from build123d import *

# Parameters (mm, degrees)
F0_W     = 1422.4
F0_H     = 50.8
F1_DEPTH = 50.8
F2_T     = -2.54


with BuildPart() as f1:
    # F0 (on Right) → F1 (new body)
    with BuildSketch(Plane.YZ):
        Rectangle(F0_W, F0_H)
    extrude(amount=F1_DEPTH)

    # F2
    f2_openings = [f1.faces().sort_by_distance(p)[0] for p in [
        (25.4, 711.2, 0),
        (25.4, -711.2, 0),
    ]]
    offset(amount=F2_T, openings=f2_openings)


solid = f1.part
Geometry: final body of the model. Coordinates: model frame, mm. A direction names the side the tool comes from. Coordinates: 2 decimals unless noted, no trailing zeros. Order: outer loops, then holes, each group sorted by start corner. A loop starts at its lowest first (then second) coordinate and runs counter-clockwise, first axis right, second up.
(1) Section query C-C (y = 340). Return the cut outline in (x, z), plus the area to 3 significant figures.
(2) Section query B-B (x = 39.5). Return the cut outline in (y, z), plus the area to 3 significant figures.
(3) First-contact query: pin 1 (6 mm diameter, centred on y = 24.5, z = 4.5, fed in from -X). Flat tip, straight axial feed; report the tip coordinate or a pass-through.
(4) Section query A-A (z = -9). Return the cut outline in (x, y).
(5) Draft query along Z for faces 3 (the face through (25, -10, 25.4)), 4 (the face through (25, -10, -25.4)), 5 (the face through (0, -10, 0)), 6 (the face through (48.26, -10, 0)). Return one class per face: pulls with the +Z half, pulls with the -Z half, needs draft (parallel to the pull), parting line crosses it, or undercut.
(6) Material intervals for probe 1 along X at (y, z) = (-635.5, -11); probe 2 along Z at (x, y) = (5, -48), sorted ascending.
(7) Access query for faces 1 (the face through (50.8, -10, 0)), 2 (the face through (25, -10, -22.86)). Directions: +Z, -Z, +X, -X, +Y, -Y. A direction counts if a zero-diameter tool reaches every point of the face in a straight line with its end or side. Return the directions, or none.
Solution:
1. outline: (0, -25.4) - (50.8, -25.4) - (50.8, 25.4) - (0, 25.4) - close; hole (2.54, -22.86) - (48.26, -22.86) - (48.26, 22.86) - (2.54, 22.86) - close
1. area: 490 mm2
2. outline: (-711.2, -25.4) - (711.2, -25.4) - (711.2, -22.86) - (-711.2, -22.86) - close; (-711.2, 22.86) - (711.2, 22.86) - (711.2, 25.4) - (-711.2, 25.4) - close
2. area: 7,230 mm2
3. pin 1: stops at x = 0
4. outline: (0, -711.2) - (2.54, -711.2) - (2.54, 711.2) - (0, 711.2) - close; (48.26, -711.2) - (50.8, -711.2) - (50.8, 711.2) - (48.26, 711.2) - close
5. face 3: pulls with the +Z half
5. face 4: pulls with the -Z half
5. face 5: needs draft
5. face 6: undercut
6. probe 1: x = 0 to 2.54, 48.26 to 50.8
6. probe 2: z = -25.4 to -22.86, 22.86 to 25.4
7. face 1: +Z, -Z, +X, +Y, -Y
7. face 2: +Y, -Y
